Here's how the part is built. I have some questions about the finished solid (model axes, mm). Face numbers are marked on the shaded views. A direction names the side the tool comes from. Coordinates: 2 decimals unless noted, no trailing zeros. Write each loop counter-clockwise with the first axis right and the second up, starting at its lowest first coordinate (ties: lowest second). Pieces come first, ordered by that corner, then holes. Notation, with made-up numbers: M 20.5,74 L 50.5,74 A13 ccw 50.5,99 Z; hole C 20,61.25 d6. An arc over 180 degrees is marked long. Use a Markdown table: item, result.
```python
from build123d import *

# Parameters (mm, degrees)
F0_R     = 6.35
F1_DEPTH = 25.4
F3_DEPTH = 25.4


with BuildPart() as f1:
    # F0 (on Front) → F1 (new body)
    with BuildSketch(Plane.XZ):
        with BuildLine():
            Line((0, 25.4), (0, 0))
            Line((0, 0), (76.2, 0))
            Line((76.2, 0), (76.2, 12.7))
            Line((76.2, 12.7), (25.4, 12.7))
            Line((25.4, 12.7), (25.4, 25.4))
            Line((25.4, 25.4), (25.4, 26.4084818092))
            ThreePointArc((25.4, 26.4084818092), (22.7211091646, 33.7222732658), (16.2787873612, 38.1))
            Line((16.2787873612, 38.1), (9.1212126388, 38.1))
            ThreePointArc((9.1212126388, 38.1), (2.6788908354, 33.7222732658), (0, 26.4084818092))
            Line((0, 26.4084818092), (0, 25.4))
        make_face()
        with Locations((12.7, 25.4)):
            Circle(F0_R, mode=Mode.SUBTRACT)
        with BuildLine():
            ThreePointArc((0, 26.4084818092), (-0.0100062506, 25.9042409046), (0, 25.4))
            Line((0, 25.4), (0, 26.4084818092))
        make_face()
        with BuildLine():
            ThreePointArc((16.2787873612, 38.1), (12.7, 38.6142471552), (9.1212126388, 38.1))
            Line((9.1212126388, 38.1), (16.2787873612, 38.1))
        make_face()
        with BuildLine():
            Line((25.4, 26.4084818092), (25.4, 25.4))
            ThreePointArc((25.4, 25.4), (25.4100062506, 25.9042409046), (25.4, 26.4084818092))
        make_face()
    extrude(amount=F1_DEPTH)

    # F2 (on face) → F3 (join)
    with BuildSketch(Plane.XY.offset(12.7)):
        with BuildLine():
            ThreePointArc((45.3922208286, -18.9798098827), (49.2621954374, -16.8438963443), (50.8006859977, -12.7))
            ThreePointArc((50.8006859977, -12.7), (49.5316727855, -8.8913160721), (46.2318440252, -6.6049219791))
            ThreePointArc((46.2318440252, -6.6049219791), (38.1152517777, -12.2701474168), (45.3922208286, -18.9798098827))
        make_face()
        with BuildLine():
            ThreePointArc((69.8506859977, -12.8319995129), (67.9747841458, -8.325898564), (63.4554274902, -6.482160801))
            ThreePointArc((63.4554274902, -6.482160801), (57.1506990788, -12.8191103921), (63.4296503294, -19.1816021724))
            ThreePointArc((63.4296503294, -19.1816021724), (67.9656285229, -17.3471726266), (69.8506859977, -12.8319995129))
        make_face()
        with BuildLine():
            ThreePointArc((46.2318440252, -6.6049219791), (49.5316727855, -8.8913160721), (50.8006859977, -12.7))
            ThreePointArc((50.8006859977, -12.7), (49.2621954374, -16.8438963443), (45.3922208286, -18.9798098827))
            Line((45.3922208286, -18.9798098827), (63.4296503294, -19.1816021724))
            ThreePointArc((63.4296503294, -19.1816021724), (57.1506990788, -12.8191103921), (63.4554274902, -6.482160801))
            Line((63.4554274902, -6.482160801), (46.2318440252, -6.6049219791))
        make_face()
    extrude(amount=F3_DEPTH)


solid = f1.part
```
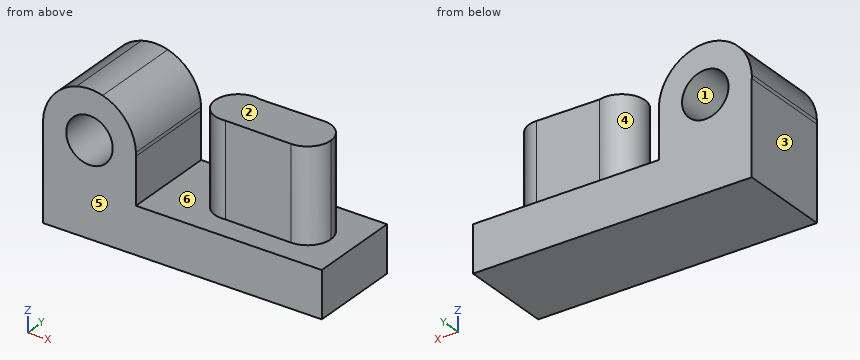
1. Which directions (+Z, -Z, +X, -X, +Y, -Y) give clear straight access to the entire face, cutting with the end or side of a thin tool? Please do the marked faces 5 and 6.
Answers follow:
| item | result |
|---|---|
| face 5 | +Z, -Z, +X, -X, -Y |
| face 6 | +Z |
2. Suppose I cut it at A-A on z = 16. Write out the boundary of the cut face in (x, y).
Answers follow:
| item | result |
|---|---|
| outline | M 0,-25.4 L 25.4,-25.4 L 25.4,0 L 0,0 Z; M 45.39,-18.98 L 63.43,-19.18 A6.35 ccw long 63.46,-6.48 L 46.23,-6.6 A6.35 ccw long Z |
3. We'd pull the mould along X, two halves only. Please class the marked faces 1, 2, 3 and 4: +X half, -X half, draft (parallel to the pull), parting line (faces both ways), or undercut.
Answers follow:
| item | result |
|---|---|
| face 1 | undercut |
| face 2 | draft |
| face 3 | -X half |
| face 4 | undercut |
4. I need wall thicknesses on probe 1 along Z at (x, y) = (12.7, -10); probe 2 along Z at (x, y) = (26, -18.75); probe 3 along X at (y, z) = (-2.75, 4.5). Which ranges of each line are inside material? Lowest first, please.
Answers follow:
| item | result |
|---|---|
| probe 1 | z = 0 to 19.05, 31.75 to 38.61 |
| probe 2 | z = 0 to 12.7 |
| probe 3 | x = 0 to 76.2 |
5. Suppose I cut it at B-B on x = 12.7. Write out the boundary of the cut face in (y, z), and give its area (3 significant figures).
Answers follow:
| item | result |
|---|---|
| outline | M -25.4,0 L 0,0 L 0,19.05 L -25.4,19.05 Z; M -25.4,31.75 L 0,31.75 L 0,38.61 L -25.4,38.61 Z |
| area | 658 mm2 |
6. Will these pins go through, and if not, where does the flat tip stop? pin 1 Ø1.5 at (x, z) = (59, 18) entering from -Y; pin 2 Ø12.5 at (x, y) = (42.5, -12) entering from +Z; pin 3 Ø10 at (y, z) = (-8.5, 33) entering from +X; pin 4 Ø1 at (x, z) = (37.5, 28.5) entering from -Y.
Answers follow:
| item | result |
|---|---|
| pin 1 | stops at y = -19.14 |
| pin 2 | stops at z = 38.1 |
| pin 3 | stops at x = 69.85 |
| pin 4 | passes through |
7. Suppose I cut it at C-C on y = -3. Write out the boundary of the cut face in (x, z), and give its area (3 significant figures).
Answers follow:
| item | result |
|---|---|
| outline | M 0,0 L 76.2,0 L 76.2,12.7 L 25.4,12.7 L 25.4,25.4 A12.71 ccw long 0,25.4 Z; hole C 12.7,25.4 d12.7 |
| area | 1,430 mm2 |
8. Suppose I cut it at D-D on z = 29. Write out the boundary of the cut face in (x, y), and give its area (3 significant figures).
Answers follow:
| item | result |
|---|---|
| outline | M 0.37,-25.4 L 7.47,-25.4 L 7.47,0 L 0.37,0 Z; M 17.93,-25.4 L 25.03,-25.4 L 25.03,0 L 17.93,0 Z; M 45.39,-18.98 L 63.43,-19.18 A6.35 ccw long 63.46,-6.48 L 46.23,-6.6 A6.35 ccw long Z |
| area | 726 mm2 |
